The listing builds one solid part. Answer for the finished solid, in the listing's coordinates (mm). A direction names the side the tool comes from. Coordinates: 2 decimals unless noted, no trailing zeros. Order: outer loops, then holes, each group sorted by start corner. A loop starts at its lowest first (then second) coordinate and runs counter-clockwise, first axis right, second up.
```python
from build123d import *

# Parameters (mm, degrees)
F0_R     = 9.95
F1_DEPTH = 70
F0_R_2   = 12.45
F2_DEPTH = 15
F0_R_3   = 14.5
F3_DEPTH = 3
F5_DEPTH = 20
F8_DEPTH = 3.95
F9_R     = 0.5


with BuildPart() as f1:
    # F0 (on Front) → F1 (new body)
    with BuildSketch(Plane.XZ):
        Circle(F0_R)
    extrude(amount=F1_DEPTH)

    # F0 (on Front) → F2 (join)
    with BuildSketch(Plane.XZ):
        Circle(F0_R_2)
        Circle(F0_R, mode=Mode.SUBTRACT)
        Circle(F0_R)
    extrude(amount=-F2_DEPTH)

    # F0 (on Front) → F3 (join)
    with BuildSketch(Plane.XZ):
        Circle(F0_R_3)
        Circle(F0_R_2, mode=Mode.SUBTRACT)
        Circle(F0_R_2)
        Circle(F0_R, mode=Mode.SUBTRACT)
        Circle(F0_R)
    extrude(amount=-F3_DEPTH)

    # F4 (on Front) → F5 (join)
    with BuildSketch(Plane.XZ):
        with BuildLine():
            Line((8.6518402555, -4.9140777561), (11.1170168717, -5.7150621934))
            ThreePointArc((11.1170168717, -5.7150621934), (11.8882064537, -3.8627124297), (12.3530848492, -1.9108361283))
            Line((12.3530848492, -1.9108361283), (9.887908233, -1.109851691))
            ThreePointArc((9.887908233, -1.109851691), (9.4630123371, -3.074719094), (8.6518402555, -4.9140777561))
        make_face()
        with BuildLine():
            Line((4.1110633656, -9.0609965238), (5.6346263027, -11.1580010051))
            ThreePointArc((5.6346263027, -11.1580010051), (7.3473156537, -10.1127124297), (8.8706942802, -8.8068599959))
            Line((8.8706942802, -8.8068599959), (7.3471313431, -6.7098555146))
            ThreePointArc((7.3471313431, -6.7098555146), (5.8484632603, -8.049719094), (4.1110633656, -9.0609965238))
        make_face()
        with BuildLine():
            ThreePointArc((2, -9.7469225913), (0, -9.95), (-2, -9.7469225913))
            Line((-2, -9.7469225913), (-2, -12.3389626793))
            ThreePointArc((-2, -12.3389626793), (0, -12.5), (2, -12.3389626793))
            Line((2, -12.3389626793), (2, -9.7469225913))
        make_face()
        with BuildLine():
            Line((-7.3471313431, -6.7098555146), (-8.8706942802, -8.8068599959))
            ThreePointArc((-8.8706942802, -8.8068599959), (-7.3473156537, -10.1127124297), (-5.6346263027, -11.1580010051))
            Line((-5.6346263027, -11.1580010051), (-4.1110633656, -9.0609965238))
            ThreePointArc((-4.1110633656, -9.0609965238), (-5.8484632603, -8.049719094), (-7.3471313431, -6.7098555146))
        make_face()
        with BuildLine():
            Line((-9.887908233, -1.109851691), (-12.3530848492, -1.9108361283))
            ThreePointArc((-12.3530848492, -1.9108361283), (-11.8882064537, -3.8627124297), (-11.1170168717, -5.7150621934))
            Line((-11.1170168717, -5.7150621934), (-8.6518402555, -4.9140777561))
            ThreePointArc((-8.6518402555, -4.9140777561), (-9.4630123371, -3.074719094), (-9.887908233, -1.109851691))
        make_face()
        with BuildLine():
            Line((-8.6518402555, 4.9140777561), (-11.1170168717, 5.7150621934))
            ThreePointArc((-11.1170168717, 5.7150621934), (-11.8882064537, 3.8627124297), (-12.3530848492, 1.9108361283))
            Line((-12.3530848492, 1.9108361283), (-9.887908233, 1.109851691))
            ThreePointArc((-9.887908233, 1.109851691), (-9.4630123371, 3.074719094), (-8.6518402555, 4.9140777561))
        make_face()
        with BuildLine():
            Line((-4.1110633656, 9.0609965238), (-5.6346263027, 11.1580010051))
            ThreePointArc((-5.6346263027, 11.1580010051), (-7.3473156537, 10.1127124297), (-8.8706942802, 8.8068599959))
            Line((-8.8706942802, 8.8068599959), (-7.3471313431, 6.7098555146))
            ThreePointArc((-7.3471313431, 6.7098555146), (-5.8484632603, 8.049719094), (-4.1110633656, 9.0609965238))
        make_face()
        with BuildLine():
            ThreePointArc((-2, 9.7469225913), (0, 9.95), (2, 9.7469225913))
            Line((2, 9.7469225913), (2, 12.3389626793))
            ThreePointArc((2, 12.3389626793), (0, 12.5), (-2, 12.3389626793))
            Line((-2, 12.3389626793), (-2, 9.7469225913))
        make_face()
        with BuildLine():
            Line((7.3471313431, 6.7098555146), (8.8706942802, 8.8068599959))
            ThreePointArc((8.8706942802, 8.8068599959), (7.3473156537, 10.1127124297), (5.6346263027, 11.1580010051))
            Line((5.6346263027, 11.1580010051), (4.1110633656, 9.0609965238))
            ThreePointArc((4.1110633656, 9.0609965238), (5.8484632603, 8.049719094), (7.3471313431, 6.7098555146))
        make_face()
        with BuildLine():
            Line((9.887908233, 1.109851691), (12.3530848492, 1.9108361283))
            ThreePointArc((12.3530848492, 1.9108361283), (11.8882064537, 3.8627124297), (11.1170168717, 5.7150621934))
            Line((11.1170168717, 5.7150621934), (8.6518402555, 4.9140777561))
            ThreePointArc((8.6518402555, 4.9140777561), (9.4630123371, 3.074719094), (9.887908233, 1.109851691))
        make_face()
    extrude(amount=F5_DEPTH)

    # F7 (on offset) → F8 (cut)
    with BuildSketch(Plane.XY.offset(6)):
        with BuildLine():
            Line((-3, -73.1982216239), (0, -73.1982216239))
            Line((0, -73.1982216239), (3, -73.1982216239))
            Line((3, -73.1982216239), (3, -53.1982216239))
            ThreePointArc((3, -53.1982216239), (0, -50.1982216239), (-3, -53.1982216239))
            Line((-3, -53.1982216239), (-3, -73.1982216239))
        make_face()
    extrude(amount=F8_DEPTH, mode=Mode.SUBTRACT)

    # F9
    f9_edges = [f1.edges().sort_by_distance(p)[0] for p in [
        (-5.880157, -70, -8.026596),
        (-3, -61.599111, 9.486965),
        (0, -50.198222, 9.95),
        (3, -61.599111, 9.486965),
    ]]
    fillet(f9_edges, radius=F9_R)


solid = f1.part
```
(1) Find section A-A (y = -58.5). Write down the section's boundary in (x, z), and give its area (3 significant figures).
(2) The mould has two halves that part along X. Classify faces 1 (the face through (0, -9.9, 12.5)), 2 (the face through (-9.87, -9.86, 5.31)), 3 (the face through (6, -20, -9)): released by +X, released by -X, zero draft, split by the parting line, or undercut.
(3) Consider line 1 (Y direction, x = 13, z = -0.5); line 2 (Z direction, x = 8, y = -14); line 3 (Y direction, x = -12, z = -0.25). Determine where each line is inside the solid, lowest interval first.
(4) Each of these flat-tipped pins is pushed along its axis until it touches: pin 1 Ø1.5 at (x, y) = (-7, -28.5) entering from +Z; pin 2 Ø4 at (x, z) = (10.5, -3) entering from -Y; pin 3 Ø1.4 at (y, z) = (-59, 7.5) entering from -X; pin 4 Ø1.5 at (x, y) = (-1.5, -3) entering from +Z. Where does it stop, or does it pass through?
(5) For faces 4 (the face through (-11, -20, -3)), 5 (the face through (-7, -20, 9)), 6 (the face through (-8.098, -9.86, -7.744)), 7 (the face through (0, -60, 6)), 8 (the face through (10, -20, -3)), determine the directions among +Z, -Z, +X, -X, +Y, -Y from which every point of the face is accessible in a straight line to the end or side of a thin tool.
(6) Find section B-B (y = 5.5). Write down the section's boundary in (x, z), and give its area (3 significant figures).
Findings below:
1. outline: (-3.69, 9.24) arc R9.95 ccw (long way) to (3.69, 9.24) arc R0.5 ccw to (3, 8.78) - (3, 6) - (-3, 6) - (-3, 8.78) arc R0.5 ccw to start
1. area: 288 mm2
2. face 1: split by the parting line
2. face 2: undercut
2. face 3: zero draft
3. line 1: y = 0 to 3
3. line 2: z = -9.6 to -7.61, -5.92 to 5.92, 7.61 to 9.6
3. line 3: y = 0 to 15
4. pin 1: stops at z = 7.74
4. pin 2: stops at y = -70
4. pin 3: stops at x = -7.26
4. pin 4: stops at z = 12.48
5. face 4: -Z, -X, -Y
5. face 5: +Z, -X, -Y
5. face 6: -X, -Y
5. face 7: +Z, -Y
5. face 8: -Z, +X, -Y
6. outline: circle Ø24.9 at (0, 0)
6. area: 487 mm2
